Geometry check sheet. Reference: the model listing, model coordinates, mm. A direction names the side the tool comes from. Coordinates: 2 decimals unless noted, no trailing zeros. Loops run counter-clockwise (first coordinate to the right, second up) from the corner with the lowest first, then second, coordinate; pieces in that order, holes last.
from build123d import *

# Parameters (mm, degrees)
F0_W     = 12.7
F0_H     = 25.4
F1_DEPTH = 6.35
F3_DEPTH = 254
F4_W     = 6.35
F4_H     = 12.7
F5_DEPTH = 254
F8_DEPTH = 25374.6


with BuildPart() as f1:
    # F0 (on Front) → F1 (new body)
    with BuildSketch(Plane.XZ):
        with Locations((-6.35, 12.7)):
            Rectangle(F0_W, F0_H)
    extrude(amount=F1_DEPTH)

    # F2 (on face) → F3 (cut)
    with BuildSketch(Plane.XZ.offset(6.35)):
        with BuildLine():
            Line((-12.7, 25.4), (-12.7, 19.05))
            ThreePointArc((-12.7, 19.05), (-10.8401280605, 23.5401280605), (-6.35, 25.4))
            Line((-6.35, 25.4), (-12.7, 25.4))
        make_face()
        with BuildLine():
            Line((0, 25.4), (-6.35, 25.4))
            ThreePointArc((-6.35, 25.4), (-1.8598719395, 23.5401280605), (0, 19.05))
            Line((0, 19.05), (0, 25.4))
        make_face()
        with BuildLine():
            ThreePointArc((0, 6.35), (-1.8598719395, 1.8598719395), (-6.35, 0))
            Line((-6.35, 0), (0, 0))
            Line((0, 0), (0, 6.35))
        make_face()
        with BuildLine():
            ThreePointArc((-6.35, 0), (-10.8401280605, 1.8598719395), (-12.7, 6.35))
            Line((-12.7, 6.35), (-12.7, 0))
            Line((-12.7, 0), (-6.35, 0))
        make_face()
    extrude(amount=-F3_DEPTH, mode=Mode.SUBTRACT)

    # F4 (on face) → F5 (cut)
    with BuildSketch(Plane.XZ.offset(6.35)):
        with BuildLine():
            Line((-8.8261451244, 19.05), (-2.4761451244, 19.05))
            ThreePointArc((-2.4761451244, 19.05), (-5.6511451244, 22.225), (-8.8261451244, 19.05))
        make_face()
        with Locations((-5.6511451244, 12.7)):
            Rectangle(F4_W, F4_H)
        with BuildLine():
            ThreePointArc((-8.8261451244, 6.35), (-5.6511451244, 3.175), (-2.4761451244, 6.35))
            Line((-2.4761451244, 6.35), (-8.8261451244, 6.35))
        make_face()
    extrude(amount=-F5_DEPTH, mode=Mode.SUBTRACT)

    # F6: F1 across plane


with BuildPart() as f1_1:
    add(f1.part)
    add(f1.part.mirror(Plane.YZ))

    # F7 (on face) → F8 (cut)
    with BuildSketch(Plane.XZ.offset(6.35)):
        with BuildLine():
            Line((0, 6.35), (0, 19.05))
            ThreePointArc((0, 19.05), (-6.35, 25.4), (-12.7, 19.05))
            Line((-12.7, 19.05), (-12.7, 6.35))
            ThreePointArc((-12.7, 6.35), (-6.35, 0), (0, 6.35))
        make_face()
        with BuildLine():
            Line((-8.8261451244, 6.35), (-8.8261451244, 19.05))
            ThreePointArc((-8.8261451244, 19.05), (-5.6511451244, 22.225), (-2.4761451244, 19.05))
            Line((-2.4761451244, 19.05), (-2.4761451244, 6.35))
            ThreePointArc((-2.4761451244, 6.35), (-5.6511451244, 3.175), (-8.8261451244, 6.35))
        make_face(mode=Mode.SUBTRACT)
    extrude(amount=-F8_DEPTH, mode=Mode.SUBTRACT)


solid = f1_1.part
1) Depth check by flat-ended pin: pin 1 (1 mm diameter, centred on x = 9, y = -2.5, fed in from +Z); pin 2 (1.5 mm diameter, centred on x = 9.5, y = -4, fed in from -Z). Enter the tip coordinate at first touch or a pass-through.
Data:
pin 1: stops at z = 25.02
pin 2: stops at z = 0.47
2) Section check C-C on x = 5. Record the cut outline in (y, z), and give its area (3 significant figures).
Data:
outline: (-6.35, 0.15) - (0, 0.15) - (0, 3.24) - (-6.35, 3.24) - close; (-6.35, 22.16) - (0, 22.16) - (0, 25.25) - (-6.35, 25.25) - close
area: 39.3 mm2
3) Access from +Z, -Z, +X, -X, +Y, -Y to the whole of each face (thin tool, end or side, straight path). Record for faces 4 (the flat face through (12.7, -3, 13)), 5 (the flat face through (8.826, -3, 13)).
Data:
face 4: +Z, -Z, +X, +Y, -Y
face 5: +Y, -Y
4) Mould release check, pull along Z, two halves, no side actions. Record for faces 1 (the cylindrical face through (5.721, -3.219, 3.176)), 2 (the flat face through (0, -3, 13)), 3 (the cylindrical face through (5.581, -3.219, 22.224)): +Z half, -Z half, draft (parallel to the pull), parting line (faces both ways), or undercut.
Data:
face 1: undercut
face 2: draft
face 3: undercut
5) Section check B-B on y = -4.75. Record the cut outline in (x, z) (3 decimals).
Data:
outline: (0, 6.35) arc R6.35 ccw to (12.7, 6.35) - (12.7, 19.05) arc R6.35 ccw to (0, 19.05) - close; hole (2.476, 6.35) arc R3.175 ccw to (8.826, 6.35) - (8.826, 19.05) arc R3.175 ccw to (2.476, 19.05) - close
6) Material ranges on probe 1 along X at (y, z) = (-2, 6.5); probe 2 along X at (y, z) = (-4, 20.25); probe 3 along Z at (x, y) = (3.5, -3.25), recorded low to high.
Data:
probe 1: x = 0 to 2.48, 8.83 to 12.7
probe 2: x = 0.11 to 2.71, 8.59 to 12.59
probe 3: z = 0.68 to 4.01, 21.39 to 24.72
7) Section check A-A on z = 18.75. Record the cut outline in (x, y).
Data:
outline: (0, -6.35) - (2.48, -6.35) - (2.48, 0) - (0, 0) - close; (8.83, -6.35) - (12.7, -6.35) - (12.7, 0) - (8.83, 0) - close
8) Section check D-D on x = 1.75. Record the cut outline in (y, z), and give its area (3 significant figures).
Data:
outline: (-6.35, 1.97) - (0, 1.97) - (0, 23.43) - (-6.35, 23.43) - close
area: 136 mm2
